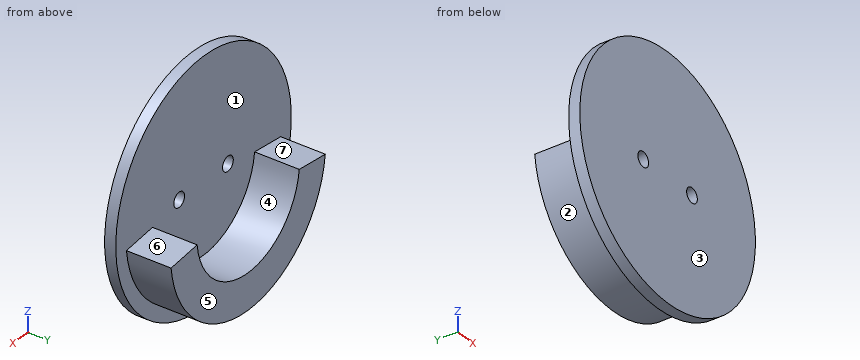
```python
from build123d import *

# Parameters (mm, degrees)
BOSS_EXTRUDE1_DEPTH = 10
SKETCH2_R           = 27
BOSS_EXTRUDE2_DEPTH = 2.5
SKETCH3_R           = 1.65
CUT_EXTRUDE1_DEPTH  = 10


with BuildPart() as part:
    # Sketch1 → Boss-Extrude1 (new body)
    with BuildSketch(Plane(origin=(0, 0, 0), x_dir=(1, 0, 0), z_dir=(0, 1, 0))):
        with BuildLine():
            Line((-23.711759029, 2.564173113), (-15.708418979, 1.698697492))
            ThreePointArc((-15.708418979, 1.698697492), (0, 15.8), (15.708418979, 1.698697492))
            Line((15.708418979, 1.698697492), (23.711759029, 2.564173113))
            ThreePointArc((23.711759029, 2.564173113), (0, 23.85), (-23.711759029, 2.564173113))
        make_face()
    extrude(amount=BOSS_EXTRUDE1_DEPTH)

    # Sketch2 → Boss-Extrude2 (add)
    with BuildSketch(Plane.XZ):
        with Locations(Location((0, 0, 0), (0, 0, 270))):
            Circle(SKETCH2_R)
    extrude(amount=BOSS_EXTRUDE2_DEPTH)

    # Sketch3 → Cut-Extrude1 (cut)
    with BuildSketch(Plane(origin=(0, 0, 0), x_dir=(1, 0, 0), z_dir=(0, 1, 0))):
        with Locations(Location((-7.5, 0, 0), (0, 0, 270))):
            Circle(SKETCH3_R)
        with Locations(Location((7.5, 0, 0), (0, 0, 90))):
            Circle(SKETCH3_R)
    extrude(amount=-CUT_EXTRUDE1_DEPTH, mode=Mode.SUBTRACT)


solid = part.part
```
Could you check a few things on this model? Use its own coordinates, in mm. Face numbers are marked on the shaded views. A direction names the side the tool comes from. Coordinates: 2 decimals unless noted, no trailing zeros. Order: outer loops, then holes, each group sorted by start corner. A loop starts at its lowest first (then second) coordinate and runs counter-clockwise, first axis right, second up. Notation, with made-up numbers: M 56.25,37.25 L 96.25,37.25 A17 cw 96.25,48.25 Z; hole C 1.25,-33.75 d6. An arc over 180 degrees is marked long. Use one line per item in the form item = value. Start each with the question number.
1. We'd pull the mould along X, two halves only. Please class the marked faces 1, 2, 3 and 4: +X half, -X half, draft (parallel to the pull), parting line (faces both ways), or undercut.
2. Suppose I cut it at A-A on z = 0. Write out the boundary of the cut face in (x, y), then the cut area to 4 significant figures.
3. Suppose I cut it at C-C on x = 7.5. Write out the boundary of the cut face in (y, z).
4. On a 3-axis mill with a long thin cutter (end or side, diameter ignored), from which of +Z, -Z, +X, -X, +Y, -Y can I reach the whole of each face in a straight line? I mean the marked faces 5, 6 and 7. Say none if no direction works.
5. Suppose I cut it at D-D on y = 7.5. Write out the boundary of the cut face in (x, z).
6. Suppose I cut it at B-B on x = 0. Write out the boundary of the cut face in (y, z), then the cut area to 4 significant figures.
7. For pin 1 (2 mm diameter, centred on x = 14, y = 2.5, fed in from -Z); pin 2 (1 mm diameter, centred on x = -1, y = 5.5, fed in from +Z); pin 3 (5 mm diameter, centred on x = -10, y = 4, fed in from +Z); pin 4 (2.5 mm diameter, centred on x = -7.5, z = 0, fed in from +Y), each with a flat end and sliding along its axis, tell me the tip position at first contact or that it passes through.
8. Please list where these lines run through material, in increasing order: line 1 (X direction, y = -0.9, z = 0); line 2 (Y direction, x = 8.5, z = -8.5); line 3 (X direction, y = 5.25, z = -13.5).
Geometry says:
q1.face_1 = undercut
q1.face_2 = parting line
q1.face_3 = draft
q1.face_4 = undercut
q2.outline = M -27,-2.5 L -9.15,-2.5 L -9.15,0 L -27,0 Z; M -5.85,-2.5 L 5.85,-2.5 L 5.85,0 L -5.85,0 Z; M 9.15,-2.5 L 27,-2.5 L 27,0 L 9.15,0 Z
q2.area = 118.5 mm^2
q3.outline = M -2.5,-25.94 L 0,-25.94 L 0,-22.64 L 10,-22.64 L 10,-13.91 L 0,-13.91 L 0,-1.65 L -2.5,-1.65 Z; M -2.5,1.65 L 0,1.65 L 0,25.94 L -2.5,25.94 Z
q4.face_5 = +Z, -Z, +X, -X, +Y
q4.face_6 = +Z, +X, +Y
q4.face_7 = +Z, -X, +Y
q5.outline = M -23.71,-2.56 A23.85 ccw 23.71,-2.56 L 15.71,-1.7 A15.8 cw -15.71,-1.7 Z
q6.outline = M -2.5,-27 L 0,-27 L 0,-23.85 L 10,-23.85 L 10,-15.8 L 0,-15.8 L 0,27 L -2.5,27 Z
q6.area = 215.5 mm^2
q7.pin_1 = -20
q7.pin_2 = -15.73
q7.pin_3 = -9.66
q7.pin_4 = through
q8.line_1 = -27 to -9.15, -5.85 to 5.85, 9.15 to 27
q8.line_2 = -2.5 to 0
q8.line_3 = -19.66 to -8.21, 8.21 to 19.66
